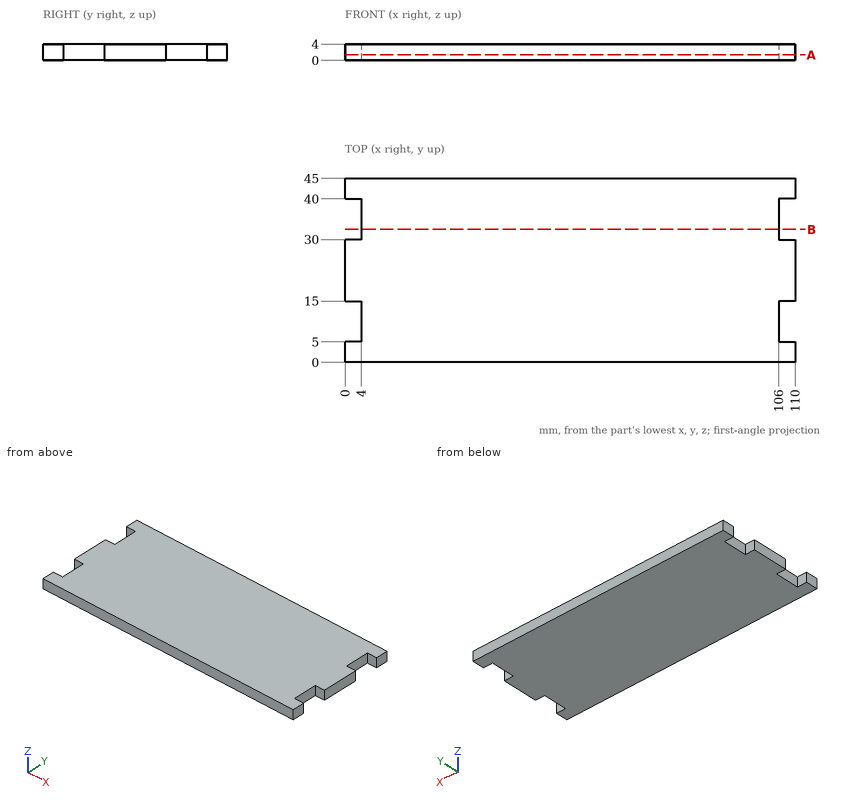
Can you work these out from the drawing? Everything is in mm from the part's minimum corner. Coordinates: 2 decimals unless noted, no trailing zeros. Loops run counter-clockwise (first coordinate to the right, second up) from the corner with the lowest first, then second, coordinate; pieces in that order, holes last. Notation, with made-up numbers: (16.25, -27.75) -> (24.25, -27.75) arc R22 cw to (24.25, -13.75) -> close; hole circle Ø7 at (-23.75, -10.5). An arc over 180 degrees is marked (long way). Return JSON: item names as keys, results as strings.
1) If we section it at B-B, the plane y = 32.5: Write out the boundary of the cut face in (x, z), then the cut area to 3 significant figures.
Results below:
{"outline": "(4, 0) -> (106, 0) -> (106, 4) -> (4, 4) -> close", "area": "408 mm²"}
2) Will these pins go through, and if not, where does the flat tip stop? pin 1 (1.2 mm diameter, centred on y = 33.5, z = 2, fed in from +X); pin 2 (1.2 mm diameter, centred on y = 12.5, z = 2.5, fed in from -X).
Results below:
{"pin 1": "x = 106", "pin 2": "x = 4"}
3) If we section it at A-A, the plane z = 1.35: Write out the boundary of the cut face in (x, y), then the cut area to 3 significant figures.
Results below:
{"outline": "(0, 0) -> (110, 0) -> (110, 5) -> (106, 5) -> (106, 15) -> (110, 15) -> (110, 30) -> (106, 30) -> (106, 40) -> (110, 40) -> (110, 45) -> (0, 45) -> (0, 40) -> (4, 40) -> (4, 30) -> (0, 30) -> (0, 15) -> (4, 15) -> (4, 5) -> (0, 5) -> close", "area": "4,790 mm²"}
4) I need wall thicknesses on line 1 (X direction, y = 31, z = 0.35). Which ranges of the line are inside material? Lowest first, please. Write a range as from..to.
Results below:
{"line 1": "4..106"}
